```python
from build123d import *

# Parameters (mm, degrees)
SKETCH1_W           = 95
SKETCH1_H           = 120
SKETCH1_R           = 1.7
BOSS_EXTRUDE1_DEPTH = 3
FILLET1_R           = 3
CUT_EXTRUDE1_DEPTH  = 10
SKETCH3_W           = 8
SKETCH3_H           = 20
CUT_EXTRUDE2_DEPTH  = 4
FILLET2_R           = 3


with BuildPart() as part:
    # Sketch1 → Boss-Extrude1 (new body)
    with BuildSketch(Plane.XY):
        with Locations((47.5, -60)):
            Rectangle(SKETCH1_W, SKETCH1_H)
        with Locations((10, -105)):
            Circle(SKETCH1_R, mode=Mode.SUBTRACT)
        with Locations((80, -110)):
            Circle(SKETCH1_R, mode=Mode.SUBTRACT)
        with Locations((10, -30)):
            Circle(SKETCH1_R, mode=Mode.SUBTRACT)
        with BuildLine():
            Line((56.109241719, -63.05462086), (66.109241719, -43.05462086))
            ThreePointArc((66.109241719, -43.05462086), (70.999425204, -40.766366896), (74.35, -45))
            ThreePointArc((74.35, -45), (74.233633104, -45.999425204), (73.890758281, -46.94537914))
            Line((73.890758281, -46.94537914), (63.890758281, -66.94537914))
            ThreePointArc((63.890758281, -66.94537914), (58.05462086, -68.890758281), (56.109241719, -63.05462086))
        make_face(mode=Mode.SUBTRACT)
    extrude(amount=BOSS_EXTRUDE1_DEPTH)

    # Fillet1
    fillet1_edges = [part.edges().sort_by_distance(p)[0] for p in [
        (0, -120, 1.5),
        (0, 0, 1.5),
        (95, 0, 1.5),
        (95, -120, 1.5),
    ]]
    fillet(fillet1_edges, radius=FILLET1_R)

    # Sketch2 → Cut-Extrude1 (cut)
    with BuildSketch(Plane.XY.offset(3)):
        with BuildLine():
            Line((30.8, -10), (30.8, -20))
            ThreePointArc((30.8, -20), (32.5, -21.7), (34.2, -20))
            Line((34.2, -20), (34.2, -10))
            ThreePointArc((34.2, -10), (32.5, -8.3), (30.8, -10))
        make_face()
        with BuildLine():
            Line((60.8, -10), (60.8, -20))
            ThreePointArc((60.8, -20), (62.5, -21.7), (64.2, -20))
            Line((64.2, -20), (64.2, -10))
            ThreePointArc((64.2, -10), (62.5, -8.3), (60.8, -10))
        make_face()
    extrude(amount=-CUT_EXTRUDE1_DEPTH, mode=Mode.SUBTRACT)

    # Sketch3 → Cut-Extrude2 (cut, through all)
    with BuildSketch(Plane.XY.offset(3)):
        with Locations((91, -110)):
            Rectangle(SKETCH3_W, SKETCH3_H)
    extrude(amount=-CUT_EXTRUDE2_DEPTH, mode=Mode.SUBTRACT)

    # Fillet2
    fillet2_edges = [part.edges().sort_by_distance(p)[0] for p in [
        (95, -100, 1.5),
        (87, -120, 1.5),
        (87, -100, 1.5),
    ]]
    fillet(fillet2_edges, radius=FILLET2_R)


solid = part.part
```
Work out the finished part from the listing and answer in its coordinate system (mm). A direction names the side the tool comes from. Give positions to 0.01 mm unless a question says otherwise; leave off trailing zeros. Loops run counter-clockwise (first coordinate to the right, second up) from the corner with the lowest first, then second, coordinate; pieces in that order, holes last. Notation, with made-up numbers: (-37.75, -12.75) -> (-0.75, -12.75) arc R23 ccw to (-0.75, 5.25) -> close; hole circle Ø5 at (-1, -22.75). An arc over 180 degrees is marked (long way). Put each result on its own line as item: value. Start each with the question number.
Item 1: Which of the six approach directions +Z, -Z, +X, -X, +Y, -Y give full straight-line access (tool end or side, diameter ignored) to faces 1 (the face through (47, -59, 0)), 2 (the face through (32.5, -8.3, 1.5)), 3 (the face through (87, -110, 2))?
Item 2: The part is cut by section B-B (x = 80). Give the vertices of the cut face in (y, z), then the cut area to 3 significant figures.
Item 3: Each of these flat-tipped pins is pushed along its axis until it touches: P1, Ø1.6, axis at x = 91, z = 1, coming from the -Y side; P2, Ø3, axis at x = 80, y = -110, coming from the +Z side. Where does it stop, or does it pass through?
Item 4: Find the intervals of material crossed by L1, parallel to X at y = -110, z = 0.75; L2, parallel to X at y = -18.5, z = 1.95; L3, parallel to X at y = -105, z = 0.9, in increasing order. Write a range as [from, to].
Item 5: The mould has two halves that part along Y. Classify faces 4 (the face through (95, -51, 1)), 5 (the face through (32.5, -21.7, 1.5)), 6 (the face through (68.96, -56.81, 1.48)), 7 (the face through (94.14, -99.1, 1.48)): released by +Y, released by -Y, zero draft, split by the parting line, or undercut.
Item 6: The part is cut by section A-A (y = -30). Give the vertices of the cut face in (x, z).
Item 7: The part is cut by section C-C (z = 1.85). Give the vertices of the cut face in (x, y).
Item 8: The part is cut by section D-D (x = 10). Give the vertices of the cut face in (y, z), then the cut area to 3 significant figures.
Answers below:
1. face 1: -Z, +X, -X, +Y, -Y
1. face 2: +Z, -Z
1. face 3: +Z, -Z, +X, -Y
2. outline: (-120, 0) -> (-111.7, 0) -> (-111.7, 3) -> (-120, 3) -> close; (-108.3, 0) -> (0, 0) -> (0, 3) -> (-108.3, 3) -> close
2. area: 350 mm2
3. P1: y = -100
3. P2: through
4. L1: [0, 78.3], [81.7, 87]
4. L2: [0, 30.8], [34.2, 60.8], [64.2, 95]
4. L3: [0, 8.3], [11.7, 87]
5. face 4: zero draft
5. face 5: undercut
5. face 6: undercut
5. face 7: released by -Y
6. outline: (0, 0) -> (8.3, 0) -> (8.3, 3) -> (0, 3) -> close; (11.7, 0) -> (95, 0) -> (95, 3) -> (11.7, 3) -> close
7. outline: (0, -117) arc R3 ccw to (3, -120) -> (84, -120) arc R3 ccw to (87, -117) -> (87, -103) arc R3 cw to (90, -100) -> (92, -100) arc R3 ccw to (95, -97) -> (95, -3) arc R3 ccw to (92, 0) -> (3, 0) arc R3 ccw to (0, -3) -> close; hole circle Ø3.4 at (10, -105); hole circle Ø3.4 at (10, -30); hole (30.8, -20) arc R1.7 ccw to (34.2, -20) -> (34.2, -10) arc R1.7 ccw to (30.8, -10) -> close; hole (56.11, -63.05) arc R4.35 ccw to (63.89, -66.95) -> (73.89, -46.95) arc R4.35 ccw to (66.11, -43.05) -> close; hole (60.8, -20) arc R1.7 ccw to (64.2, -20) -> (64.2, -10) arc R1.7 ccw to (60.8, -10) -> close; hole circle Ø3.4 at (80, -110)
8. outline: (-120, 0) -> (-106.7, 0) -> (-106.7, 3) -> (-120, 3) -> close; (-103.3, 0) -> (-31.7, 0) -> (-31.7, 3) -> (-103.3, 3) -> close; (-28.3, 0) -> (0, 0) -> (0, 3) -> (-28.3, 3) -> close
8. area: 340 mm2
